Could you check a few things on this model? Use its own coordinates, in mm. Round coordinates to 2 decimals unless told otherwise and drop trailing zeros. Loops run counter-clockwise (first coordinate to the right, second up) from the corner with the lowest first, then second, coordinate; pieces in that order, holes last. Notation, with made-up numbers: (27.25, -34) - (39.25, -34) arc R17 cw to (39.25, -16) - close; hole circle Ø7 at (-2.5, 80). An arc over 180 degrees is marked (long way). Answer as CSV lines item,"result". Start each with the question number.
1) I'm going to push a flat-ended pin straight in: pin 1 Ø5.5 at (y, z) = (134.83, -152.87) entering from +X. Where does the tip first touch, or does it pass through?
2) Suppose I cut it at B-B, the plane z = -186. Write out the boundary of the cut face in (x, y).
3) Please list where these lines run through material, in increasing order: line 1 along Y through (x, z) = (-486.5, -153); line 2 along Z through (x, y) = (-480.75, 158.5); line 3 along Y through (x, z) = (-482.5, -184).
4) Suppose I cut it at C-C, the plane x = -486. Write out the boundary of the cut face in (y, z).
5) Suppose I cut it at A-A, the plane y = 161.5. Write out the boundary of the cut face in (x, z).
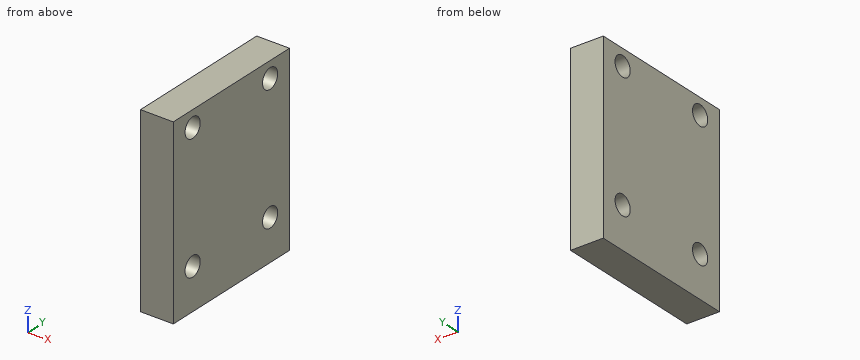
```python
from build123d import *

# Parameters (mm, degrees)
SKETCH2_W                  = 46.228
SKETCH2_H                  = 38.1
BOSS_EXTRUDE1_DEPTH        = 8.255
F_10_CLEARANCE_HOLE1_D     = 4.9784
F_10_CLEARANCE_HOLE1_DEPTH = 25.4
F_10_CLEARANCE_HOLE1_TIP   = 1.495662253


with BuildPart() as part:
    # Sketch2 → Boss-Extrude1 (new body)
    with BuildSketch(Plane(origin=(-488.965433296, 0, 0), x_dir=(0, 0, -1), z_dir=(1, 0, 0))):
        with Locations((171.873330939, 147.533779805)):
            Rectangle(SKETCH2_W, SKETCH2_H)
    extrude(amount=BOSS_EXTRUDE1_DEPTH)

    # #10 Clearance Hole1
    with Locations(Plane.ZY.offset(488.965433296)):
        with Locations((-184.616110941, 160.233779805), (-152.866110941, 160.233779805), (-152.866110941, 134.833779805), (-184.616110941, 134.833779805)):
            Hole(F_10_CLEARANCE_HOLE1_D / 2, depth=F_10_CLEARANCE_HOLE1_DEPTH)
            with Locations((0, 0, -(F_10_CLEARANCE_HOLE1_DEPTH + F_10_CLEARANCE_HOLE1_TIP / 2))):  # 118° drill point
                Cone(0, F_10_CLEARANCE_HOLE1_D / 2, F_10_CLEARANCE_HOLE1_TIP, mode=Mode.SUBTRACT)


solid = part.part
```
Filled sheet:
1,pin 1,"x = -480.71"
2,outline,"(-488.97, 128.48) - (-480.71, 128.48) - (-480.71, 132.76) - (-488.97, 132.76) - close; (-488.97, 136.9) - (-480.71, 136.9) - (-480.71, 158.16) - (-488.97, 158.16) - close; (-488.97, 162.3) - (-480.71, 162.3) - (-480.71, 166.58) - (-488.97, 166.58) - close"
3,line 1,"128.48 to 132.35, 137.32 to 157.75, 162.72 to 166.58"
3,line 2,"-194.99 to -186.4, -182.83 to -154.65, -151.08 to -148.76"
3,line 3,"128.48 to 132.42, 137.25 to 157.82, 162.65 to 166.58"
4,outline,"(128.48, -194.99) - (166.58, -194.99) - (166.58, -148.76) - (128.48, -148.76) - close; hole circle Ø4.98 at (134.83, -184.62); hole circle Ø4.98 at (134.83, -152.87); hole circle Ø4.98 at (160.23, -184.62); hole circle Ø4.98 at (160.23, -152.87)"
5,outline,"(-488.97, -194.99) - (-480.71, -194.99) - (-480.71, -186.76) - (-488.97, -186.76) - close; (-488.97, -182.47) - (-480.71, -182.47) - (-480.71, -155.01) - (-488.97, -155.01) - close; (-488.97, -150.72) - (-480.71, -150.72) - (-480.71, -148.76) - (-488.97, -148.76) - close"
